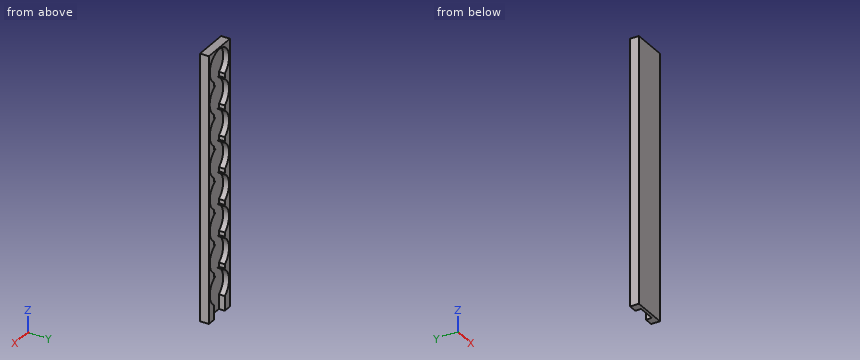
from build123d import *

# Parameters (mm, degrees)
SKETCH1_W           = 23.5
SKETCH1_H           = 181
BOSS_EXTRUDE1_DEPTH = 6
SKETCH2_R           = 10.75
CUT_EXTRUDE1_DEPTH  = 4
SKETCH3_W           = 12
SKETCH3_H           = 2.830218613
CUT_EXTRUDE2_DEPTH  = 4
SKETCH5_R           = 10.75
CUT_EXTRUDE5_DEPTH  = 4
LPATTERN1_COUNT     = 8
LPATTERN1_PITCH     = 21.49
SKETCH4_W           = 12
SKETCH4_H           = 4
CUT_EXTRUDE3_DEPTH  = 8.07


with BuildPart() as part:
    # Sketch1 → Boss-Extrude1 (new body)
    with BuildSketch(Plane(origin=(0, 0, 0), x_dir=(1, 0, 0), z_dir=(0, 1, 0))):
        with Locations((11.75, 90.5)):
            Rectangle(SKETCH1_W, SKETCH1_H)
    extrude(amount=-BOSS_EXTRUDE1_DEPTH)

    # Sketch2 → Cut-Extrude1 (cut)
    with BuildSketch(Plane(origin=(0, 0, 0), x_dir=(1, 0, 0), z_dir=(0, 1, 0))):
        with Locations((11.75, 11.75)):
            Circle(SKETCH2_R)
    cut_extrude1 = extrude(amount=-CUT_EXTRUDE1_DEPTH, mode=Mode.SUBTRACT)

    # Sketch3 → Cut-Extrude2 (cut)
    with BuildSketch(Plane(origin=(0, 0, 0), x_dir=(1, 0, 0), z_dir=(0, 1, 0))):
        with Locations((11.75, 22.084890694)):
            Rectangle(SKETCH3_W, SKETCH3_H)
    cut_extrude2 = extrude(amount=-CUT_EXTRUDE2_DEPTH, mode=Mode.SUBTRACT)

    # Sketch5 → Cut-Extrude5 (cut)
    with BuildSketch(Plane(origin=(0, 0, 0), x_dir=(1, 0, 0), z_dir=(0, 1, 0))):
        with Locations((11.845268795, 33.25)):
            Circle(SKETCH5_R)
    extrude(amount=-CUT_EXTRUDE5_DEPTH, mode=Mode.SUBTRACT)

    # LPattern1: Cut-Extrude1, Cut-Extrude2 ×8
    with Locations(*[(0, 0, -i * LPATTERN1_PITCH) for i in range(1, LPATTERN1_COUNT)]):
        add(cut_extrude1, mode=Mode.SUBTRACT)
        add(cut_extrude2, mode=Mode.SUBTRACT)

    # Sketch4 → Cut-Extrude3 (cut, through all)
    with BuildSketch(Plane.XY.offset(-173.93)):
        with Locations((11.75, -2)):
            Rectangle(SKETCH4_W, SKETCH4_H)
    extrude(amount=-CUT_EXTRUDE3_DEPTH, mode=Mode.SUBTRACT)


solid = part.part
CAD build for the part. Positions are in the model's coordinates, mm. Give positions to 0.01 mm unless a question says otherwise; leave off trailing zeros. Order: outer loops, then holes, each group sorted by start corner. A loop starts at its lowest first (then second) coordinate and runs counter-clockwise, first axis right, second up. Notation, with made-up numbers: (81, -36) -> (125, -36) arc R21 ccw to (125, -18) -> close; hole circle Ø7 at (71.25, -1). An arc over 180 degrees is marked (long way). Return JSON: item names as keys, results as strings.
Q1. Saw through at C-C (z = -30.5). Write the cut outline in (x, y).
Working result:
{"outline": "(0, -6) -> (23.5, -6) -> (23.5, 0) -> (22.24, 0) -> (22.24, -4) -> (1.36, -4) -> (1.36, 0) -> (0, 0) -> close"}
Q2. Flat gauge pins, fed straight in: pin 1 (1.5 mm diameter, centred on x = 9, y = -2, fed in from -Z); pin 2 (1 mm diameter, centred on x = 10, z = -93.5, fed in from +Y). Where does each tip first touch, or does it go through?
Working result:
{"pin 1": "z = -1.59", "pin 2": "y = -4"}
Q3. Saw through at A-A (z = -11.75). Write the cut outline in (x, y), then the cut area to 3 significant figures.
Working result:
{"outline": "(0, -6) -> (23.5, -6) -> (23.5, 0) -> (22.5, 0) -> (22.5, -4) -> (1, -4) -> (1, 0) -> (0, 0) -> close", "area": "55.0 mm²"}
Q4. Saw through at B-B (x = 11.75). Write the cut outline in (y, z).
Working result:
{"outline": "(-6, -181) -> (-4, -181) -> (-4, -1) -> (0, -1) -> (0, 0) -> (-6, 0) -> close"}
Q5. Drill centre lines: line 1 (X direction, y = -0.9, z = -11.75); line 2 (Y direction, x = 11.25, z = -158); line 3 (X direction, y = -0.7, z = -149). Where is each one in solid material? Low to high.
Working result:
{"line 1": "0 to 1, 22.5 to 23.5", "line 2": "-6 to -4", "line 3": "0 to 4.93, 18.57 to 23.5"}
